Read the model definition and answer for the solid it produces. Units are mm, in the model's axes. Give positions to 0.01 mm unless a question says otherwise; leave off trailing zeros. Order: outer loops, then holes, each group sorted by start corner. A loop starts at its lowest first (then second) coordinate and runs counter-clockwise, first axis right, second up. Notation, with made-up numbers: (45.25, 7.5) - (58.25, 7.5) arc R36 ccw to (58.25, 41.5) - close; hole circle Ø3 at (-25.5, -37). An arc over 180 degrees is marked (long way). Use a Markdown table: item, result. Add a question column.
1. A cutting plane is placed at B-B on x = -19.5. Determine the outline of the cut face in (y, z), and give its area (3 significant figures).
2. Consider L1, parallel to Y at x = -3.5, z = 0.15; L2, parallel to Y at x = -19, z = 0.2; L3, parallel to X at y = 4, z = 0.1. Determine where each line is inside the solid, lowest interval first.
3. A cutting plane is placed at C-C on x = 26. Determine the outline of the cut face in (y, z), and give its area (3 significant figures).
4. A cutting plane is placed at A-A on y = -9. Determine the outline of the cut face in (x, z), and give its area (3 significant figures).
5. A flat-ended cylindrical pin translates along its axis: P1, Ø6, axis at x = -30, y = 4.5, coming from the -Z side. Find the tip coordinate at first contact, or state that the pin passes through.
6. A cutting plane is placed at D-D on z = 0.2. State how many separate pieces and enclosed holes the cut face has, and give its area (3 significant figures).
```python
from build123d import *

# Parameters (mm, degrees)
SKETCH4_R           = 42.545
BOSS_EXTRUDE2_DEPTH = 0.254
SKETCH5_R           = 29.845
CUT_EXTRUDE5_DEPTH  = 1.254
SKETCH6_R           = 4.699
CUT_EXTRUDE6_DEPTH  = 1.254
CUT_EXTRUDE11_DEPTH = 1.254


with BuildPart() as part:
    # Sketch4 → Boss-Extrude2 (new body)
    with BuildSketch(Plane.XY):
        Circle(SKETCH4_R)
    extrude(amount=BOSS_EXTRUDE2_DEPTH)

    # Sketch5 → Cut-Extrude5 (cut, through all)
    with BuildSketch(Plane.XY.offset(0.254)):
        Circle(SKETCH5_R)
    extrude(amount=-CUT_EXTRUDE5_DEPTH, mode=Mode.SUBTRACT)

    # Sketch6 → Cut-Extrude6 (cut, through all)
    with BuildSketch(Plane.XY.offset(0.254)):
        with Locations((36.195, 0)):
            Circle(SKETCH6_R)
        with BuildLine():
            ThreePointArc((28.916424148, -28.916425271), (28.916424774, -22.271035245), (22.271034748, -22.271035613))
            ThreePointArc((22.271034748, -22.271035613), (12.052997339, -29.098509775), (5.1e-07, -31.496))
            ThreePointArc((5.1e-07, -31.496), (-4.699, -36.195000076), (6.62e-07, -40.894))
            ThreePointArc((6.62e-07, -40.894), (15.649456222, -37.781129628), (28.916424148, -28.916425271))
        make_face()
        with BuildLine():
            ThreePointArc((-28.916425271, -28.916424148), (-22.271035245, -28.916424774), (-22.271035613, -22.271034748))
            ThreePointArc((-22.271035613, -22.271034748), (-29.098509775, -12.052997339), (-31.496, -5.1e-07))
            ThreePointArc((-31.496, -5.1e-07), (-36.195000076, 4.699), (-40.894, -6.62e-07))
            ThreePointArc((-40.894, -6.62e-07), (-37.781129628, -15.649456222), (-28.916425271, -28.916424148))
        make_face()
        with BuildLine():
            ThreePointArc((-28.916424148, 28.916425271), (-28.916424774, 22.271035245), (-22.271034748, 22.271035613))
            ThreePointArc((-22.271034748, 22.271035613), (-12.052997339, 29.098509775), (-5.1e-07, 31.496))
            ThreePointArc((-5.1e-07, 31.496), (4.699, 36.195000076), (-6.62e-07, 40.894))
            ThreePointArc((-6.62e-07, 40.894), (-15.649456222, 37.781129628), (-28.916424148, 28.916425271))
        make_face()
    extrude(amount=-CUT_EXTRUDE6_DEPTH, mode=Mode.SUBTRACT)

    # Sketch8 → Cut-Extrude11 (cut, through all)
    with BuildSketch(Plane.XY.offset(0.254)):
        with BuildLine():
            Line((39.205799167, 14.864935644), (38.282384044, 17.094256956))
            Line((38.282384044, 17.094256956), (27.115548897, 12.468802389))
            ThreePointArc((27.115548897, 12.468802389), (21.103601885, 21.103601885), (12.468802389, 27.115548897))
            Line((12.468802389, 27.115548897), (17.094256956, 38.282384044))
            Line((17.094256956, 38.282384044), (14.864935644, 39.205799167))
            Line((14.864935644, 39.205799167), (15.107939624, 39.79246267))
            Line((15.107939624, 39.79246267), (16.28126663, 39.306454711))
            ThreePointArc((16.28126663, 39.306454711), (30.083858006, 30.083858006), (39.306454711, 16.28126663))
            Line((39.306454711, 16.28126663), (39.79246267, 15.107939624))
            Line((39.79246267, 15.107939624), (39.205799167, 14.864935644))
        make_face()
        Polygon((-15.350943603, 40.379126173), (-17.697597616, 39.407110255), (-17.211589657, 38.233783248), (-14.864935644, 39.205799167), align=None)
        Polygon((-39.407110255, 17.697597616), (-40.379126173, 15.350943603), (-39.205799167, 14.864935644), (-38.233783248, 17.211589657), align=None)
        Polygon((-40.379126173, -15.350943603), (-39.407110255, -17.697597616), (-38.233783248, -17.211589657), (-39.205799167, -14.864935644), align=None)
        Polygon((-17.697597616, -39.407110255), (-15.350943603, -40.379126173), (-14.864935644, -39.205799167), (-17.211589657, -38.233783248), align=None)
        Polygon((15.350943603, -40.379126173), (17.697597616, -39.407110255), (17.211589657, -38.233783248), (14.864935644, -39.205799167), align=None)
        Polygon((39.407110255, -17.697597616), (40.379126173, -15.350943603), (39.205799167, -14.864935644), (38.233783248, -17.211589657), align=None)
    extrude(amount=-CUT_EXTRUDE11_DEPTH, mode=Mode.SUBTRACT)


solid = part.part
```
Output values:
| question | item | result |
|---|---|---|
| 1 | outline | (-37.81, 0) - (-22.59, 0) - (-22.59, 0.25) - (-37.81, 0.25) - close; (22.59, 0) - (24.73, 0) - (24.73, 0.25) - (22.59, 0.25) - close; (35.95, 0) - (37.81, 0) - (37.81, 0.25) - (35.95, 0.25) - close |
| 1 | area | 4.88 mm² |
| 2 | L1 | -42.4 to -39.33, -33.06 to -29.64, 29.64 to 31.3, 40.74 to 42.4 |
| 2 | L2 | -38.07 to -23.02, 23.02 to 25.12, 36.21 to 38.07 |
| 2 | L3 | -42.36 to -38.66, -33.73 to -29.58, 29.58 to 33.73, 38.66 to 42.36 |
| 3 | outline | (-33.68, 0) - (-31.56, 0) - (-31.56, 0.25) - (-33.68, 0.25) - close; (-20.91, 0) - (-14.65, 0) - (-14.65, 0.25) - (-20.91, 0.25) - close |
| 3 | area | 2.13 mm² |
| 4 | outline | (-41.58, 0) - (-39.89, 0) - (-39.89, 0.25) - (-41.58, 0.25) - close; (-30.18, 0) - (-28.46, 0) - (-28.46, 0.25) - (-30.18, 0.25) - close; (28.46, 0) - (41.58, 0) - (41.58, 0.25) - (28.46, 0.25) - close |
| 4 | area | 4.20 mm² |
| 5 | P1 | z = 0 |
| 6 | separate pieces | 1 |
| 6 | enclosed holes | 4 |
| 6 | area | 1,460 mm² |
